CAD build for the part. Positions are in the model's coordinates, mm. A direction names the side the tool comes from. Coordinates: 2 decimals unless noted, no trailing zeros. Loops run counter-clockwise (first coordinate to the right, second up) from the corner with the lowest first, then second, coordinate; pieces in that order, holes last. Notation, with made-up numbers: (-16, 27.25) - (2, 27.25) arc R26 cw to (2, 66.25) - close; hole circle Ø1 at (60, -16). An arc over 180 degrees is marked (long way). Put each result on its own line as item: value.
```python
from build123d import *

# Parameters (mm, degrees)
F0_W      = 71.5
F0_H      = 32
F1_DEPTH  = 30.5
F3_DEPTH  = 35.75
F4_W      = 12
F4_H      = 33.5
F5_DEPTH  = 35.75
F7_DEPTH  = 80
F8_R      = 2
F9_T      = -1.6
F10_W     = 23
F10_H     = 14
F11_DEPTH = 25


with BuildPart() as f1:
    # F0 (on Top) → F1 (new body)
    with BuildSketch(Plane.XY):
        Rectangle(F0_W, F0_H)
    extrude(amount=F1_DEPTH)

    # F2 (on Right) → F3 (join, symmetric)
    with BuildSketch(Plane.YZ):
        Polygon((-16, 30.5), (0, 30.5), (16, 30.5), (16, 46.5), (-6, 46.5), align=None)
    extrude(amount=F3_DEPTH, both=True)

    # F4 (on Right) → F5 (join, symmetric)
    with BuildSketch(Plane.YZ):
        with Locations((10, 63.25)):
            Rectangle(F4_W, F4_H)
    extrude(amount=F5_DEPTH, both=True)

    # F6 (on Top) → F7 (join)
    with BuildSketch(Plane.XY):
        Polygon((-7.75, -2), (0, 4), (0, 16), (-35.75, 16), (-35.75, -2), align=None)
    extrude(amount=F7_DEPTH)

    # F8
    f8_edges = [f1.edges().sort_by_distance(p)[0] for p in [
        (0, 4, 63.25),
        (-7.75, -2, 63.25),
        (17.875, 4, 46.5),
        (0, -6, 46.5),
        (0, -16, 30.5),
        (35.75, 4, 63.25),
        (35.75, 16, 40),
        (0, 16, 80),
        (35.75, 10, 80),
        (17.875, 4, 80),
        (-21.75, -2, 80),
        (-35.75, 7, 80),
        (-35.75, -2, 63.25),
        (-35.75, 16, 40),
        (-35.75, -11, 38.5),
        (-35.75, -16, 15.25),
        (-35.75, -4, 46.5),
        (35.75, -11, 38.5),
        (35.75, -16, 15.25),
        (-21.75, -2, 46.5),
        (35.75, -1, 46.5),
        (-3.875, 1, 46.5),
        (-3.875, 1, 80),
    ]]
    fillet(f8_edges, radius=F8_R)

    # F9
    f9_openings = [f1.faces().sort_by_distance(p)[0] for p in [
        (0, 0, 0),
    ]]
    offset(amount=F9_T, openings=f9_openings)


with BuildPart() as f11:
    # F10 (on Front) → F11 (new body)
    with BuildSketch(Plane.XZ):
        Rectangle(F10_W, F10_H)
    extrude(amount=F11_DEPTH)


with BuildPart() as f1_1:
    add(f1.part)

    # F12: cut F11
    add(f11.part, mode=Mode.SUBTRACT)


solid = f1_1.part
```
Q1. Mould opens along Y. For faces 4 (the cylindrical face through (35.15, -1.49, 45.93)), 5 (the cylindrical face through (-35.18, -15.4, 15.17)), 6 (the flat face through (34.15, 3, 31)) say: +Y half, -Y half, draft (parallel to the pull), parting line (faces both ways), or undercut.
Determined:
face 4: draft
face 5: -Y half
face 6: undercut
Q2. Slice it at D-D, the plane z = 61.5. Give the cut face in (x, y).
Determined:
outline: (-35.75, 0) arc R2 ccw to (-33.75, -2) - (-8.43, -2) arc R2 ccw to (-7.21, -1.58) - (-0.54, 3.58) arc R2 cw to (0.68, 4) - (33.75, 4) arc R2 ccw to (35.75, 6) - (35.75, 14) arc R2 ccw to (33.75, 16) - (-33.75, 16) arc R2 ccw to (-35.75, 14) - close; hole (-34.15, 0) arc R0.4 ccw to (-33.75, -0.4) - (-8.43, -0.4) arc R0.4 ccw to (-8.19, -0.32) - (-1.52, 4.85) arc R3.6 cw to (0.68, 5.6) - (33.75, 5.6) arc R0.4 ccw to (34.15, 6) - (34.15, 14) arc R0.4 ccw to (33.75, 14.4) - (-33.75, 14.4) arc R0.4 ccw to (-34.15, 14) - close
Q3. Tool access for faces 1 (the flat face through (0, -14.4, 15)), 2 (the flat face through (17, 4, 63)), 3 (the flat face through (0.473, -11.078, 38.375)): list every direction of +Z, -Z, +X, -X, +Y, -Y with a clear straight run to the whole face (end or side of a thin tool).
Determined:
face 1: -Z
face 2: +Z, +X, -Y
face 3: +Z, +X, -X, -Y
Q4. Slice it at A-A, the plane z = 20.5. Give the cut face in (x, y), then the cut area to 3 significant figures.
Determined:
outline: (-35.75, -14) arc R2 ccw to (-33.75, -16) - (33.75, -16) arc R2 ccw to (35.75, -14) - (35.75, 14) arc R2 ccw to (33.75, 16) - (-33.75, 16) arc R2 ccw to (-35.75, 14) - close; hole (-34.15, -14) arc R0.4 ccw to (-33.75, -14.4) - (33.75, -14.4) arc R0.4 ccw to (34.15, -14) - (34.15, 14) arc R0.4 ccw to (33.75, 14.4) - (-33.75, 14.4) arc R0.4 ccw to (-34.15, 14) - close
area: 318 mm2
Q5. Slice it at B-B, the plane x = 5. Give the cut face in (y, z), then the cut area to 3 significant figures.
Determined:
outline: (-16, 7) - (-14.4, 7) - (-14.4, 29.93) arc R0.4 cw to (-14.34, 30.14) - (-5.23, 44.71) arc R0.4 cw to (-4.89, 44.9) - (2, 44.9) arc R3.6 ccw to (5.6, 48.5) - (5.6, 78) arc R0.4 cw to (6, 78.4) - (14, 78.4) arc R0.4 cw to (14.4, 78) - (14.4, 0) - (16, 0) - (16, 78) arc R2 ccw to (14, 80) - (6, 80) arc R2 ccw to (4, 78) - (4, 48.5) arc R2 cw to (2, 46.5) - (-4.89, 46.5) arc R2 ccw to (-6.59, 45.56) - (-15.7, 30.99) arc R2 ccw to (-16, 29.93) - close
area: 276 mm2
Q6. Wall check: L1, parallel to Y at x = -23.5, z = 22.5; L2, parallel to X at y = 12, z = 37.5; L3, parallel to Z at x = 6, y = 2. Give the ranges that are in metal, low to high. Write a range as from..to.
Determined:
L1: -16..-14.4, 14.4..16
L2: -35.75..-34.15, 34.15..35.75
L3: 44.9..46.5
Q7. Slice it at C-C, the plane y = 13. Give the cut face in (x, z).
Determined:
outline: (-35.75, 0) - (-34.15, 0) - (-34.15, 78) arc R0.4 cw to (-33.75, 78.4) - (33.75, 78.4) arc R0.4 cw to (34.15, 78) - (34.15, 0) - (35.75, 0) - (35.75, 78) arc R2 ccw to (33.75, 80) - (-33.75, 80) arc R2 ccw to (-35.75, 78) - close
Q8. Pin check, flat tips, straight feed: pin 1 Ø6 at (x, y) = (14.5, 3.5) entering from -Z; pin 2 Ø15 at (x, z) = (16.5, 66.5) entering from -Y; pin 3 Ø1.3 at (y, z) = (-15.5, 3.5) entering from +X; pin 4 Ø12 at (y, z) = (-13, 71) entering from +X. Stop position of each tip, or through.
Determined:
pin 1: z = 44.9
pin 2: y = 4
pin 3: x = 35.56
pin 4: through
